Geometry check sheet. Reference: the model listing, model coordinates, mm. A direction names the side the tool comes from. Coordinates: 2 decimals unless noted, no trailing zeros. Write each loop counter-clockwise with the first axis right and the second up, starting at its lowest first coordinate (ties: lowest second). Pieces come first, ordered by that corner, then holes. Notation, with made-up numbers: (-11.5, 80) -> (44.5, 80) arc R24 ccw to (44.5, 111) -> close; hole circle Ø7 at (13, 62). An arc over 180 degrees is marked (long way). Use a Markdown table: item, result.
```python
from build123d import *

# Parameters (mm, degrees)
F0_R     = 5
F1_DEPTH = 40
F2_R     = 5
F3_DEPTH = 10
F5_DEPTH = 15


with BuildPart() as f1:
    # F0 (on Front) → F1 (new body)
    with BuildSketch(Plane.XZ):
        with BuildLine():
            Line((-23.440344, 48.342409), (-32.454428, 48.342409))
            Line((-32.454428, 48.342409), (-32.454428, 8.342409))
            Line((-32.454428, 8.342409), (47.545572, 8.342409))
            Line((47.545572, 8.342409), (47.545572, 48.342409))
            Line((47.545572, 48.342409), (31.944597, 48.342409))
            ThreePointArc((31.944597, 48.342409), (4.252126, 29.880481), (-23.440344, 48.342409))
        make_face()
        with Locations((-22.454428, 18.342409)):
            Circle(F0_R, mode=Mode.SUBTRACT)
        with Locations((37.545572, 18.342409)):
            Circle(F0_R, mode=Mode.SUBTRACT)
    extrude(amount=F1_DEPTH)

    # F2 (on face) → F3 (cut)
    with BuildSketch(Plane.XZ.offset(40)):
        with BuildLine():
            ThreePointArc((31.944597, 48.342409), (22.240368, 35.871666), (7.545572, 30.061809))
            Line((7.545572, 30.061809), (7.545572, 8.342409))
            Line((7.545572, 8.342409), (47.545572, 8.342409))
            Line((47.545572, 8.342409), (47.545572, 48.342409))
            Line((47.545572, 48.342409), (31.944597, 48.342409))
        make_face()
        with Locations((37.545572, 18.342409)):
            Circle(F2_R, mode=Mode.SUBTRACT)
    extrude(amount=-F3_DEPTH, mode=Mode.SUBTRACT)

    # F4 (on face) → F5 (cut)
    with BuildSketch(Plane.XZ.offset(40)):
        Polygon((-32.454428, 34.042006), (-10.991666, 34.042006), (-23.440344, 48.342409), (-32.454428, 48.342409), align=None)
    extrude(amount=-F5_DEPTH, mode=Mode.SUBTRACT)


solid = f1.part
```
Item 1: Section check B-B on z = 22. Record the boundary of the cut face in (x, y).
Answer block:
| item | result |
|---|---|
| outline | (-32.45, -40) -> (-25.86, -40) -> (-25.86, 0) -> (-32.45, 0) -> close; (-19.05, -40) -> (7.55, -40) -> (7.55, -30) -> (34.14, -30) -> (34.14, 0) -> (-19.05, 0) -> close; (40.95, -30) -> (47.55, -30) -> (47.55, 0) -> (40.95, 0) -> close |
Item 2: Mould release check, pull along X, two halves, no side actions. Record for faces 4 (the flat face through (47.546, -15, 28)), 5 (the cylindrical face through (32.55, -14.79, 18.56)), 6 (the flat face through (40, -15, 48.342)), 7 (the cylindrical face through (4.746, -15.276, 29.885)): +X half, -X half, draft (parallel to the pull), parting line (faces both ways), or undercut.
Answer block:
| item | result |
|---|---|
| face 4 | +X half |
| face 5 | undercut |
| face 6 | draft |
| face 7 | undercut |
Item 3: Tool access check on faces 1 (the flat face through (-24, -25, 40)), 2 (the flat face through (7, -20, 8.342)), 3 (the flat face through (7.546, -35, 19)). Record the directions out of +Z, -Z, +X, -X, +Y, -Y that give a thin tool (end or side, any length) a straight path to the whole face; none if there is none.
Answer block:
| item | result |
|---|---|
| face 1 | +Z, -X, -Y |
| face 2 | -Z, +X, -X, +Y, -Y |
| face 3 | +Z, -Z, +X, -Y |
Item 4: Section check D-D on z = 41.5. Record the boundary of the cut face in (x, y), then the cut area to 3 significant figures.
Answer block:
| item | result |
|---|---|
| outline | (-32.45, -25) -> (-19.46, -25) -> (-19.46, 0) -> (-32.45, 0) -> close; (27.96, -30) -> (47.55, -30) -> (47.55, 0) -> (27.96, 0) -> close |
| area | 912 mm^2 |
Item 5: Thickness scan on L1, parallel to Y at x = 41, z = 45; L2, parallel to X at y = -12, z = 36; L3, parallel to X at y = -36.5, z = 12.5. Record the ranges inside material, lowest first. Write a range as [from, to].
Answer block:
| item | result |
|---|---|
| L1 | y = [-30, 0] |
| L2 | x = [-32.45, -13.91], [22.41, 47.55] |
| L3 | x = [-32.45, 7.55] |
Item 6: Section check A-A on y = -28. Record the boundary of the cut face in (x, z), then the cut area to 3 significant figures.
Answer block:
| item | result |
|---|---|
| outline | (-32.45, 8.34) -> (47.55, 8.34) -> (47.55, 48.34) -> (31.94, 48.34) arc R30 cw to (-10.99, 34.04) -> (-32.45, 34.04) -> close; hole circle Ø10 at (-22.45, 18.34); hole circle Ø10 at (37.55, 18.34) |
| area | 2,110 mm^2 |
Item 7: Section check C-C on x = -20. Record the boundary of the cut face in (y, z), then the cut area to 3 significant figures.
Answer block:
| item | result |
|---|---|
| outline | (-40, 8.34) -> (0, 8.34) -> (0, 13.99) -> (-40, 13.99) -> close; (-40, 22.7) -> (0, 22.7) -> (0, 42.22) -> (-25, 42.22) -> (-25, 34.04) -> (-40, 34.04) -> close |
| area | 884 mm^2 |
Item 8: Depth check by flat-ended pin: P1, Ø5, axis at y = -28, z = 38.5, coming from the -X side; P2, Ø7, axis at x = -25, z = 40.5, coming from the -Y side; P3, Ø3, axis at y = -35.5, z = 19, coming from the +X side. Enter the tip coordinate at first touch or a pass-through.
Answer block:
| item | result |
|---|---|
| P1 | stops at x = 22.41 |
| P2 | stops at y = -25 |
| P3 | stops at x = 7.55 |
